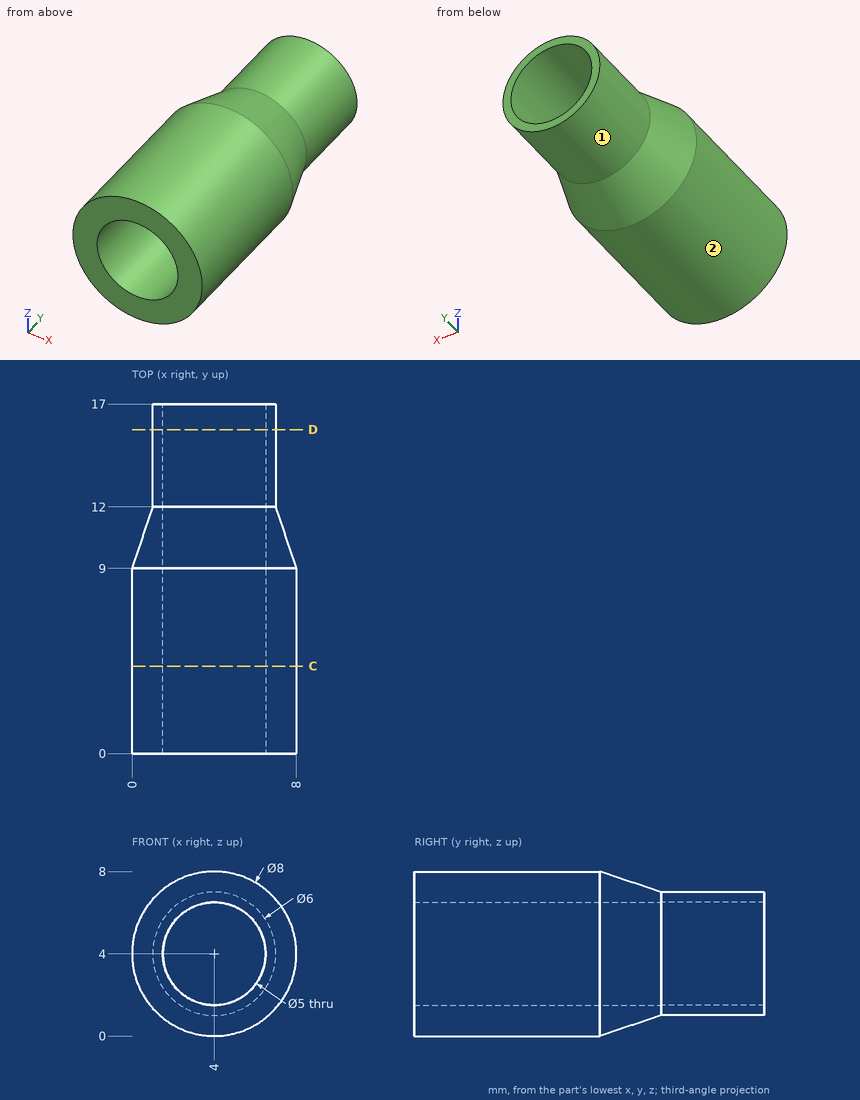
Could you check a few things on this drawing? It's one solid part, dimensions in mm from its lowest x, y, z. A direction names the side the tool comes from. Give positions to 0.01 mm unless a question says otherwise; leave off trailing zeros. Order: outer loops, then holes, each group sorted by start corner. A loop starts at its lowest first (then second) coordinate and runs counter-clockwise, first axis right, second up. Notation, with made-up numbers: (-39.5, 68) -> (9.5, 68) arc R15 ccw to (9.5, 87) -> close; hole circle Ø11 at (56.5, -36.75). An arc over 180 degrees is marked (long way). Use CSV: the item, a comma, the result in double quotes. Start each with the question number.
Item 1: Suppose I cut it at C-C (y = 4.25). List the corners of the cut face in (x, z) for me.
Item 2: If I drill on probe 1 along Z at (x, y) = (4, 15.8); probe 2 along Z at (x, y) = (4, 9); probe 3 along X at (y, z) = (10, 5.5), over which ranges is the centre line in solid material (lowest first)? Write a range as [from, to].
Item 3: Suppose I cut it at D-D (y = 15.75). List the corners of the cut face in (x, z) for me, and give its area (3 significant figures).
Item 4: On a 3-axis mill with a long thin cutter (end or side, diameter ignored), from which of +Z, -Z, +X, -X, +Y, -Y can I reach the whole of each face in a straight line? I mean the marked faces 1 and 2. Say none if no direction works.
Item 5: I'm going to push flat-ended pins straight in: P1, Ø3, axis at y = 8, z = 6, coming from the +X side; P2, Ø3, axis at y = 8.5, z = 7, coming from the -X side; P3, Ø3, axis at x = 1.5, y = 7.5, coming from the +Z side. Where does each tip first touch, or does it pass through?
Answer block:
1,outline,"circle Ø8 at (4, 4); hole circle Ø5 at (4, 4)"
2,probe 1,"z = [1, 1.5], [6.5, 7]"
2,probe 2,"z = [0, 1.5], [6.5, 8]"
2,probe 3,"x = [0.65, 2], [6, 7.35]"
3,outline,"circle Ø6 at (4, 4); hole circle Ø5 at (4, 4)"
3,area,"8.64 mm^2"
4,face 1,"+Y"
4,face 2,"+Y, -Y"
5,P1,"stops at x = 7.97"
5,P2,"stops at x = 0.29"
5,P3,"stops at z = 7.87"
